Read the model definition and answer for the solid it produces. Units are mm, in the model's axes. A direction names the side the tool comes from. Give positions to 0.01 mm unless a question says otherwise; leave off trailing zeros. Loops run counter-clockwise (first coordinate to the right, second up) from the corner with the lowest first, then second, coordinate; pieces in that order, holes last. Notation, with made-up numbers: (72.5, -37) - (105.5, -37) arc R28 ccw to (105.5, 0) - close; hole circle Ø4 at (17, 53.5). An arc over 180 degrees is marked (long way). Put each result on its own line as item: value. Start each with the question number.
1. A cutting plane is placed at D-D, the plane y = 14. Determine the outline of the cut face in (x, z).
2. A cutting plane is placed at B-B, the plane z = 0. Determine the outline of the cut face in (x, y), plus the area to 3 significant figures.
3. Consider L1, parallel to X at y = 24, z = 3.5; L2, parallel to Z at x = -5, y = 27.75; L3, parallel to Y at x = -1, z = -1.5. Determine where each line is inside the solid, lowest interval first. Write a range as from..to.
4. Given pin 1 Ø1.5 at (x, y) = (-8, 14) entering from +Z; pin 2 Ø6 at (y, z) = (11, 9.5) entering from -X; pin 3 Ø3.5 at (y, z) = (21.5, 3) entering from -X, each flat-ended and moving along its own axis, determine where each tip first touches the part or whether it passes through.
5. A cutting plane is placed at C-C, the plane x = 10.5. Determine the outline of the cut face in (y, z).
6. For a pull along X with two mould halves and no side action, classify faces 1 (the flat face through (11, 28, -3)), 2 (the cylindrical face through (-15.62, 14.79, -3.47)), 3 (the flat face through (0, 30, 10)) as released by +X, released by -X, zero draft, split by the parting line, or undercut.
7. For faces 4 (the cylindrical face through (5.828, 23.697, 4.319)), 5 (the flat face through (0, 0, 0)), determine the directions among +Z, -Z, +X, -X, +Y, -Y from which every point of the face is accessible in a straight line to the end or side of a thin tool.
8. A cutting plane is placed at A-A, the plane y = 25. Determine the outline of the cut face in (x, z).
```python
from build123d import *

# Parameters (mm, degrees)
SKETCH1_R           = 16
BOSS_EXTRUDE1_DEPTH = 30
SKETCH2_W           = 22
SKETCH2_H           = 16
CUT_EXTRUDE1_DEPTH  = 3
SKETCH3_R           = 2
CUT_EXTRUDE2_DEPTH  = 6.7
SKETCH4_W           = 22
SKETCH4_H           = 3
CUT_EXTRUDE3_DEPTH  = 8.76


with BuildPart() as part:
    # Sketch1 → Boss-Extrude1 (new body)
    with BuildSketch(Plane(origin=(0, 0, 0), x_dir=(1, 0, 0), z_dir=(0, 1, 0))):
        with Locations(Location((0, 0, 0), (0, 0, 270))):
            Circle(SKETCH1_R)
    extrude(amount=BOSS_EXTRUDE1_DEPTH)

    # Sketch2 → Cut-Extrude1 (cut)
    with BuildSketch(Plane(origin=(0, 30, 0), x_dir=(1, 0, 0), z_dir=(0, 1, 0))):
        Rectangle(SKETCH2_W, SKETCH2_H)
    extrude(amount=-CUT_EXTRUDE1_DEPTH, mode=Mode.SUBTRACT)

    # Sketch3 → Cut-Extrude2 (cut)
    with BuildSketch(Plane(origin=(0, 27, 0), x_dir=(1, 0, 0), z_dir=(0, 1, 0))):
        with Locations(Location((-7.78, -4.752687539, 0), (0, 0, 270))):
            Circle(SKETCH3_R)
        with Locations(Location((7.78, -4.752687539, 0), (0, 0, 270))):
            Circle(SKETCH3_R)
    extrude(amount=-CUT_EXTRUDE2_DEPTH, mode=Mode.SUBTRACT)

    # Sketch4 → Cut-Extrude3 (cut)
    with BuildSketch(Plane(origin=(0, 27, 0), x_dir=(1, 0, 0), z_dir=(0, 1, 0))):
        with Locations((0, 6.5)):
            Rectangle(SKETCH4_W, SKETCH4_H)
    extrude(amount=-CUT_EXTRUDE3_DEPTH, mode=Mode.SUBTRACT)


solid = part.part
```
Return value:
1. outline: circle Ø32 at (0, 0)
2. outline: (-16, 0) - (16, 0) - (16, 30) - (11, 30) - (11, 27) - (-11, 27) - (-11, 30) - (-16, 30) - close
2. area: 894 mm2
3. L1: x = -15.61..-9.34, -6.22..6.22, 9.34..15.61
3. L2: z = -15.2..-8, 8..15.2
3. L3: y = 0..27
4. pin 1: stops at z = 14.26
4. pin 2: stops at x = -14.62
4. pin 3: stops at x = -15.95
5. outline: (0, -12.07) - (30, -12.07) - (30, -8) - (18.24, -8) - (18.24, -5) - (27, -5) - (27, 8) - (30, 8) - (30, 12.07) - (0, 12.07) - close
6. face 1: undercut
6. face 2: split by the parting line
6. face 3: zero draft
7. face 4: +Y
7. face 5: +Z, -Z, +X, -X, -Y
8. outline: circle Ø32 at (0, 0); hole (-11, -8) - (11, -8) - (11, -5) - (-11, -5) - close; hole circle Ø4 at (-7.78, 4.75); hole circle Ø4 at (7.78, 4.75)
